from build123d import *

# Parameters (mm, degrees)
F0_R     = 80
F0_R_2   = 28
F1_DEPTH = 100
F2_R     = 10
F3_DEPTH = 250
F5_DEPTH = 100.0010001
F8_DEPTH = 50


with BuildPart() as f1:
    # F0 (on Top) → F1 (new body)
    with BuildSketch(Plane.XY):
        Circle(F0_R)
        Circle(F0_R_2, mode=Mode.SUBTRACT)
    extrude(amount=F1_DEPTH)

    # F2 (on Right) → F3 (cut, symmetric)
    with BuildSketch(Plane.YZ):
        with Locations((-50, 50)):
            Circle(F2_R)
    extrude(amount=F3_DEPTH, both=True, mode=Mode.SUBTRACT)

    # F4 (on face) → F5 (cut, through all)
    with BuildSketch(Plane.XY.offset(100)):
        with BuildLine():
            ThreePointArc((2.5, -27.8881695348), (0, -28), (-2.5, -27.8881695348))
            Line((-2.5, -27.8881695348), (-2.5, -79.9609279586))
            ThreePointArc((-2.5, -79.9609279586), (0, -80), (2.5, -79.9609279586))
            Line((2.5, -79.9609279586), (2.5, -27.8881695348))
        make_face()
    extrude(amount=-F5_DEPTH, mode=Mode.SUBTRACT)

    # F7 (on offset) → F8 (cut)
    with BuildSketch(Plane.YZ.offset(80)):
        with BuildLine():
            ThreePointArc((-50, 40), (-60, 50), (-50, 60))
            Line((-50, 60), (-70, 60))
            Line((-70, 60), (-70, 40))
            Line((-70, 40), (-50, 40))
        make_face()
    extrude(amount=-F8_DEPTH, mode=Mode.SUBTRACT)


solid = f1.part
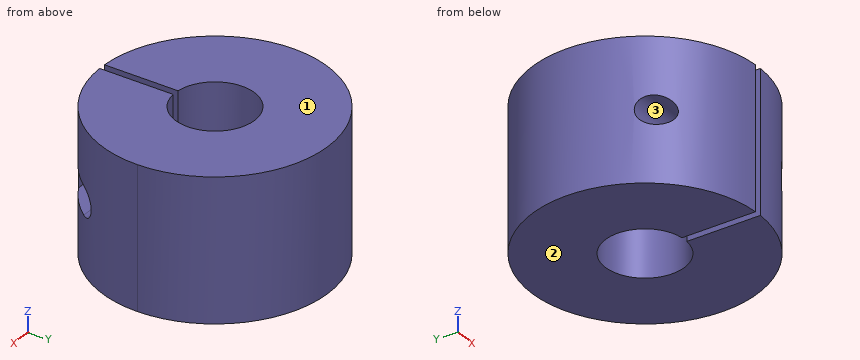
Could you check a few things on this model? Use its own coordinates, in mm. Face numbers are marked on the shaded views. Give positions to 0.01 mm unless a question says otherwise; leave off trailing zeros. Order: outer loops, then holes, each group sorted by start corner. A loop starts at its lowest first (then second) coordinate and runs counter-clockwise, first axis right, second up.
Item 1: I'm going to push flat-ended pins straight in: pin 1 (15.5 mm diameter, centred on y = -60.5, z = 35.5, fed in from -X); pin 2 (3 mm diameter, centred on x = -33, z = 26.5, fed in from +Y); pin 3 (12 mm diameter, centred on y = 13, z = 34, fed in from -X). Where does each tip first touch, or does it pass through?
Item 2: If we mould it in two halves opening along Z, with no side actions, what happens to the marked faces 1, 2 and 3? For each: pulls with the +Z half, pulls with the -Z half, needs draft (parallel to the pull), parting line crosses it, or undercut.
Item 3: If we section it at C-C, the plane x = 48: Write out the boundary of the cut face in (y, z).
Item 4: I need wall thicknesses on line 1 (Z direction, x = 37, y = -50); line 2 (Y direction, x = 11, z = 33); line 3 (X direction, y = -23, z = 90). Which ranges of each line are inside material? Lowest first, please.
Item 5: If we section it at A-A, the plane x = 17: Write out the boundary of the cut face in (y, z), plus the area to 3 significant figures.
Item 6: If we section it at D-D, the plane z = 57.5: Write out the boundary of the cut face in (x, y), plus the area to 3 significant figures.
Item 7: If we section it at B-B, the plane y = 3: Write out the boundary of the cut face in (x, z), plus the area to 3 significant figures.
Values:
1. pin 1: stops at x = -60.15
1. pin 2: stops at y = 73.54
1. pin 3: stops at x = -79.69
2. face 1: pulls with the +Z half
2. face 2: pulls with the -Z half
2. face 3: undercut
3. outline: (-64, 0) - (64, 0) - (64, 100) - (-64, 100) - (-64, 60) - (-50, 60) arc R10 cw to (-50, 40) - (-64, 40) - close
4. line 1: z = 0 to 40, 60 to 100
4. line 2: y = -79.24 to -25.75, 25.75 to 79.24
4. line 3: x = -76.62 to -15.97, 15.97 to 76.62
5. outline: (-78.17, 0) - (-22.25, 0) - (-22.25, 100) - (-78.17, 100) - close; (22.25, 0) - (78.17, 0) - (78.17, 100) - (22.25, 100) - close; hole circle Ø20 at (-50, 50)
5. area: 10,900 mm2
6. outline: (-67.21, -43.39) - (-2.5, -43.39) - (-2.5, -27.89) arc R28 cw (long way) to (2.5, -27.89) - (2.5, -43.39) - (67.21, -43.39) arc R80 ccw (long way) to start; (-56.52, -56.61) arc R80 ccw to (-2.5, -79.96) - (-2.5, -56.61) - close; (2.5, -79.96) arc R80 ccw to (38.73, -70) - (30, -70) - (30, -56.61) - (2.5, -56.61) - close
6. area: 15,600 mm2
7. outline: (-79.94, 0) - (-27.84, 0) - (-27.84, 100) - (-79.94, 100) - close; (27.84, 0) - (79.94, 0) - (79.94, 100) - (27.84, 100) - close
7. area: 10,400 mm2
